from build123d import *

# Parameters (mm, degrees)
CROQUIS1_R                 = 7.5
SALIENTE_EXTRUIR1_DEPTH    = 10
C_PULA1_FACE_RADIUS        = 7.5
C_PULA1_HEIGHT             = 7.5
CORTAR_EXTRUIR1_DEPTH      = 10
CORTAR_EXTRUIR1_DEPTH_BACK = 19
CORTAR_EXTRUIR2_DEPTH      = 11
CORTAR_EXTRUIR2_DEPTH_BACK = 19
CROQUIS3_R                 = 1.25
REDONDEO1_R                = 0.5


with BuildPart() as part:
    # Croquis1 → Saliente-Extruir1 (new body)
    with BuildSketch(Plane.XY):
        Circle(CROQUIS1_R)
    extrude(amount=SALIENTE_EXTRUIR1_DEPTH)

    # Cúpula1: a dome of height H over a round flat face of radius A is a cap of a sphere of radius (A * A + H * H) / (2 * H)
    c_pula1_r = (C_PULA1_FACE_RADIUS * C_PULA1_FACE_RADIUS + C_PULA1_HEIGHT * C_PULA1_HEIGHT) / (2 * C_PULA1_HEIGHT)
    c_pula1_base = Plane((0, 0, 10), z_dir=(0, 0, 1))
    with Locations(c_pula1_base.offset(C_PULA1_HEIGHT - c_pula1_r)):
        c_pula1_ball = Sphere(c_pula1_r, mode=Mode.PRIVATE)
    add(split(c_pula1_ball, bisect_by=c_pula1_base, keep=Keep.TOP, mode=Mode.PRIVATE))

    # Croquis2 → Cortar-Extruir1 (cut, two sides: drawn at the far end of the back side and taken through both)
    with BuildSketch(Plane(origin=(0, 0, 0), x_dir=(1, 0, 0), z_dir=(0, 1, 0)).offset(-CORTAR_EXTRUIR1_DEPTH_BACK)):
        Polygon((-4, -10), (-4, -17.5), (4, -17.5), (4, -9.5), (4, -5), (-4, -5), align=None)
    extrude(amount=CORTAR_EXTRUIR1_DEPTH + CORTAR_EXTRUIR1_DEPTH_BACK, mode=Mode.SUBTRACT)

    # Croquis3 → Cortar-Extruir2 (cut, two sides: drawn at the far end of the back side and taken through both)
    with BuildSketch(Plane(origin=(0, 0, 0), x_dir=(0, 0, -1), z_dir=(1, 0, 0)).offset(-CORTAR_EXTRUIR2_DEPTH_BACK)):
        with Locations(Location((-10, 0, 0), (0, 0, 270))):
            Circle(CROQUIS3_R)
    extrude(amount=CORTAR_EXTRUIR2_DEPTH + CORTAR_EXTRUIR2_DEPTH_BACK, mode=Mode.SUBTRACT)

    # Redondeo1
    # the kernel refuses this fillet: 0.5 mm, written as the material it takes off along each edge
    with BuildSketch(Plane(origin=(0, 0, 5), x_dir=(-0.6663010614300323, 0.7456828384354923, 0), z_dir=(-0.7456828384354923, -0.6663010614300323, 0))) as redondeo1_piece_1_section:
        with BuildLine():
            CenterArc((7.5 - REDONDEO1_R, REDONDEO1_R), REDONDEO1_R, 270, 90)
            Line((7.5 - REDONDEO1_R, 0), (7.5, 0))
            Line((7.5, 0), (7.5, REDONDEO1_R))
        make_face()
    redondeo1_piece_1 = revolve(axis=Axis((0, 0, 5), (0, 0, -1)), revolution_arc=83.564433706, mode=Mode.PRIVATE)
    redondeo1_piece_1 = split(redondeo1_piece_1, bisect_by=Plane(origin=(4, 7.359307854, 4.859307854), z_dir=(-1, 0, 0)), keep=Keep.TOP, mode=Mode.PRIVATE)
    redondeo1_piece_1 = split(redondeo1_piece_1, bisect_by=Plane(origin=(-4, 7.359307854, 4.859307854), z_dir=(1, 0, 0)), keep=Keep.TOP, mode=Mode.PRIVATE)
    add(redondeo1_piece_1, mode=Mode.SUBTRACT)
    with BuildSketch(Plane(origin=(4, -6.34428877, 10), x_dir=(0.807803952835934, 0.5894512480117758, 0), z_dir=(0, 0, -1)), Plane(origin=(-4, 6.34428877, 10), x_dir=(-0.8078039528359331, -0.5894512480117771, 0), z_dir=(0, 0, -1))) as redondeo1_piece_2:
        with BuildLine():
            CenterArc((0.982970703, -0.498849769), REDONDEO1_R, 86.112875875, 130.005200885)
            Line((0.579068726, -0.793575393), (0, 0))
            ThreePointArc((0, 0), (0.508433122, 0.017253461), (1.016866244, 0))
        make_face()
    extrude(amount=5, mode=Mode.SUBTRACT)
    with BuildSketch(Plane(origin=(4, 6.34428877, 10), x_dir=(0.8078039528359339, -0.5894512480117758, 0), z_dir=(0, 0, -1)), Plane(origin=(-4, -6.34428877, 10), x_dir=(-0.8078039528359333, 0.5894512480117767, 0), z_dir=(0, 0, -1))) as redondeo1_piece_3:
        with BuildLine():
            CenterArc((0.982970703, 0.498849769), REDONDEO1_R, 143.88192324, 130.005200885)
            Line((0.579068726, 0.793575393), (0, 0))
            ThreePointArc((0, 0), (0.508433122, -0.017253461), (1.016866244, 0))
        make_face()
    extrude(amount=5, mode=Mode.SUBTRACT)
    with BuildSketch(Plane(origin=(-4, 0, 10), x_dir=(0, 1, 0), z_dir=(0, 0, -1))) as redondeo1_piece_4:
        with BuildLine():
            CenterArc((5.361902647, -0.5), REDONDEO1_R, 319.994799115, 130.005200885)
            ThreePointArc((5.744895694, -0.821428571), (6.058529646, -0.42088436), (6.34428877, 0))
            Line((6.34428877, 0), (5.361902647, 0))
        make_face()
    revolve(axis=Axis((-4, 0, 10), (1, 0, 0)), revolution_arc=180, mode=Mode.SUBTRACT)
    with BuildSketch(Plane(origin=(4, 0, 10), x_dir=(0, 1, 0), z_dir=(0, 0, -1))) as redondeo1_piece_5:
        with BuildLine():
            CenterArc((5.361902647, 0.5), REDONDEO1_R, 270, 130.005200885)
            Line((5.361902647, 0), (6.34428877, 0))
            ThreePointArc((6.34428877, 0), (6.058529646, 0.42088436), (5.744895694, 0.821428571))
        make_face()
    revolve(axis=Axis((4, 0, 10), (1, 0, 0)), revolution_arc=180, mode=Mode.SUBTRACT)
    with BuildSketch(Plane(origin=(0, 0, 5), x_dir=(0.6663010614300334, -0.7456828384354912, 0), z_dir=(0.7456828384354912, 0.6663010614300334, 0))) as redondeo1_piece_6_section:
        with BuildLine():
            CenterArc((7.5 - REDONDEO1_R, REDONDEO1_R), REDONDEO1_R, 270, 90)
            Line((7.5 - REDONDEO1_R, 0), (7.5, 0))
            Line((7.5, 0), (7.5, REDONDEO1_R))
        make_face()
    redondeo1_piece_6 = revolve(axis=Axis((0, 0, 5), (0, 0, -1)), revolution_arc=83.564433706, mode=Mode.PRIVATE)
    redondeo1_piece_6 = split(redondeo1_piece_6, bisect_by=Plane(origin=(4, -7.359307854, 4.859307854), z_dir=(-1, 0, 0)), keep=Keep.TOP, mode=Mode.PRIVATE)
    redondeo1_piece_6 = split(redondeo1_piece_6, bisect_by=Plane(origin=(-4, -7.359307854, 4.859307854), z_dir=(1, 0, 0)), keep=Keep.TOP, mode=Mode.PRIVATE)
    add(redondeo1_piece_6, mode=Mode.SUBTRACT)
    with BuildSketch(Plane(origin=(-4, 6.34428877, 10), x_dir=(-0.8078039528359331, -0.5894512480117771, 0), z_dir=(0, 0, -1))) as redondeo1_piece_7a_section:
        with BuildLine():
            CenterArc((0.982970703, -0.498849769), REDONDEO1_R, 86.112875875, 130.005200885)
            Line((0.579068726, -0.793575393), (0, 0))
            ThreePointArc((0, 0), (0.508433122, 0.017253461), (1.016866244, 0))
        make_face()
    redondeo1_piece_7a = extrude(amount=7.54216561, mode=Mode.PRIVATE)
    redondeo1_piece_7a = split(redondeo1_piece_7a, bisect_by=Plane(origin=(-4.209576919, 5.957871406, 5), z_dir=(0, 0, -1)), keep=Keep.TOP, mode=Mode.PRIVATE)
    with BuildSketch(Plane(origin=(0, 0, 5), x_dir=(-0.6663010614300323, 0.7456828384354923, 0), z_dir=(-0.7456828384354923, -0.6663010614300323, 0))) as redondeo1_piece_7b_section:
        with BuildLine():
            CenterArc((7.5 - REDONDEO1_R, REDONDEO1_R), REDONDEO1_R, 270, 90)
            Line((7.5 - REDONDEO1_R, 0), (7.5, 0))
            Line((7.5, 0), (7.5, REDONDEO1_R))
        make_face()
    redondeo1_piece_7b = revolve(axis=Axis((0, 0, 5), (0, 0, -1)), revolution_arc=83.564433706, mode=Mode.PRIVATE)
    redondeo1_piece_7b = split(redondeo1_piece_7b, bisect_by=Plane(origin=(-4, 5.878976183, 4.882052038), z_dir=(-1, 0, 0)), keep=Keep.TOP, mode=Mode.PRIVATE)
    redondeo1_piece_7 = redondeo1_piece_7a & redondeo1_piece_7b
    add(redondeo1_piece_7, mode=Mode.SUBTRACT)
    with BuildSketch(Plane(origin=(0, 0, 5), x_dir=(-0.6663010614300323, 0.7456828384354923, 0), z_dir=(-0.7456828384354923, -0.6663010614300323, 0))) as redondeo1_piece_8a_section:
        with BuildLine():
            CenterArc((7.5 - REDONDEO1_R, REDONDEO1_R), REDONDEO1_R, 270, 90)
            Line((7.5 - REDONDEO1_R, 0), (7.5, 0))
            Line((7.5, 0), (7.5, REDONDEO1_R))
        make_face()
    redondeo1_piece_8a = revolve(axis=Axis((0, 0, 5), (0, 0, -1)), revolution_arc=83.564433706, mode=Mode.PRIVATE)
    redondeo1_piece_8a = split(redondeo1_piece_8a, bisect_by=Plane(origin=(4, 5.878976375, 4.882052003), z_dir=(1, 0, 0)), keep=Keep.TOP, mode=Mode.PRIVATE)
    with BuildSketch(Plane(origin=(4, 6.34428877, 10), x_dir=(0.8078039528359339, -0.5894512480117758, 0), z_dir=(0, 0, -1))) as redondeo1_piece_8b_section:
        with BuildLine():
            CenterArc((0.982970703, 0.498849769), REDONDEO1_R, 143.88192324, 130.005200885)
            Line((0.579068726, 0.793575393), (0, 0))
            ThreePointArc((0, 0), (0.508433122, -0.017253461), (1.016866244, 0))
        make_face()
    redondeo1_piece_8b = extrude(amount=7.54216561, mode=Mode.PRIVATE)
    redondeo1_piece_8b = split(redondeo1_piece_8b, bisect_by=Plane(origin=(4.209576919, 5.957871406, 5), z_dir=(0, 0, -1)), keep=Keep.TOP, mode=Mode.PRIVATE)
    redondeo1_piece_8 = redondeo1_piece_8a & redondeo1_piece_8b
    add(redondeo1_piece_8, mode=Mode.SUBTRACT)
    with BuildSketch(Plane(origin=(4, -6.34428877, 10), x_dir=(0.807803952835934, 0.5894512480117758, 0), z_dir=(0, 0, -1))) as redondeo1_piece_9a_section:
        with BuildLine():
            CenterArc((0.982970703, -0.498849769), REDONDEO1_R, 86.112875875, 130.005200885)
            Line((0.579068726, -0.793575393), (0, 0))
            ThreePointArc((0, 0), (0.508433122, 0.017253461), (1.016866244, 0))
        make_face()
    redondeo1_piece_9a = extrude(amount=7.54216561, mode=Mode.PRIVATE)
    redondeo1_piece_9a = split(redondeo1_piece_9a, bisect_by=Plane(origin=(4.209576919, -5.957871406, 5), z_dir=(0, 0, -1)), keep=Keep.TOP, mode=Mode.PRIVATE)
    with BuildSketch(Plane(origin=(0, 0, 5), x_dir=(0.6663010614300334, -0.7456828384354912, 0), z_dir=(0.7456828384354912, 0.6663010614300334, 0))) as redondeo1_piece_9b_section:
        with BuildLine():
            CenterArc((7.5 - REDONDEO1_R, REDONDEO1_R), REDONDEO1_R, 270, 90)
            Line((7.5 - REDONDEO1_R, 0), (7.5, 0))
            Line((7.5, 0), (7.5, REDONDEO1_R))
        make_face()
    redondeo1_piece_9b = revolve(axis=Axis((0, 0, 5), (0, 0, -1)), revolution_arc=83.564433706, mode=Mode.PRIVATE)
    redondeo1_piece_9b = split(redondeo1_piece_9b, bisect_by=Plane(origin=(4, -5.878976176, 4.88205204), z_dir=(1, 0, 0)), keep=Keep.TOP, mode=Mode.PRIVATE)
    redondeo1_piece_9 = redondeo1_piece_9a & redondeo1_piece_9b
    add(redondeo1_piece_9, mode=Mode.SUBTRACT)
    with BuildSketch(Plane(origin=(0, 0, 5), x_dir=(0.6663010614300334, -0.7456828384354912, 0), z_dir=(0.7456828384354912, 0.6663010614300334, 0))) as redondeo1_piece_10a_section:
        with BuildLine():
            CenterArc((7.5 - REDONDEO1_R, REDONDEO1_R), REDONDEO1_R, 270, 90)
            Line((7.5 - REDONDEO1_R, 0), (7.5, 0))
            Line((7.5, 0), (7.5, REDONDEO1_R))
        make_face()
    redondeo1_piece_10a = revolve(axis=Axis((0, 0, 5), (0, 0, -1)), revolution_arc=83.564433706, mode=Mode.PRIVATE)
    redondeo1_piece_10a = split(redondeo1_piece_10a, bisect_by=Plane(origin=(-4, -5.878976383, 4.882052), z_dir=(-1, 0, 0)), keep=Keep.TOP, mode=Mode.PRIVATE)
    with BuildSketch(Plane(origin=(-4, -6.34428877, 10), x_dir=(-0.8078039528359333, 0.5894512480117767, 0), z_dir=(0, 0, -1))) as redondeo1_piece_10b_section:
        with BuildLine():
            CenterArc((0.982970703, 0.498849769), REDONDEO1_R, 143.88192324, 130.005200885)
            Line((0.579068726, 0.793575393), (0, 0))
            ThreePointArc((0, 0), (0.508433122, -0.017253461), (1.016866244, 0))
        make_face()
    redondeo1_piece_10b = extrude(amount=7.54216561, mode=Mode.PRIVATE)
    redondeo1_piece_10b = split(redondeo1_piece_10b, bisect_by=Plane(origin=(-4.209576919, -5.957871406, 5), z_dir=(0, 0, -1)), keep=Keep.TOP, mode=Mode.PRIVATE)
    redondeo1_piece_10 = redondeo1_piece_10a & redondeo1_piece_10b
    add(redondeo1_piece_10, mode=Mode.SUBTRACT)


solid = part.part
The listing builds one solid part. Answer for the finished solid, in the listing's coordinates (mm). A direction names the side the tool comes from. Round coordinates to 2 decimals unless told otherwise and drop trailing zeros. Order: outer loops, then holes, each group sorted by start corner. A loop starts at its lowest first (then second) coordinate and runs counter-clockwise, first axis right, second up. Notation, with made-up numbers: (13.25, 36) -> (72.25, 36) arc R13 ccw to (72.25, 52) -> close; hole circle Ø5 at (86, 73.25). An arc over 180 degrees is marked (long way). One line per item, written item: value.
Item 1: Given P1, Ø1.5, axis at x = 6, z = 14, coming from the -Y side; P2, Ø5, axis at x = 3, z = 12, coming from the -Y side; P3, Ø2.5, axis at x = -1, y = 0.5, coming from the +Z side, each flat-ended and moving along its own axis, determine where each tip first touches the part or whether it passes through.
Taken from the geometry:
P1: stops at y = -3.81
P2: stops at y = -5.86
P3: stops at z = 5
Item 2: Find section D-D, the plane x = 0. Give the vertices of the cut face in (y, z), then the cut area to 3 significant figures.
Taken from the geometry:
outline: (-7.5, 0) -> (7.5, 0) -> (7.5, 4.5) arc R0.5 ccw to (7, 5) -> (-7, 5) arc R0.5 ccw to (-7.5, 4.5) -> close
area: 74.9 mm2
Item 3: Find section B-B, the plane y = 0. Give the vertices of the cut face in (x, z).
Taken from the geometry:
outline: (-7.5, 0) -> (7.5, 0) -> (7.5, 8.75) -> (4, 8.75) -> (4, 5) -> (-4, 5) -> (-4, 8.75) -> (-7.5, 8.75) -> close; (-7.4, 11.25) -> (-4, 11.25) -> (-4, 15.36) arc R0.5 ccw to (-4.82, 15.74) arc R7.5 ccw to start; (4, 11.25) -> (7.4, 11.25) arc R7.5 ccw to (4.82, 15.74) arc R0.5 ccw to (4, 15.36) -> close
Item 4: For a pull along X with two mould halves and no side action, classify faces 1 (the cylindrical face through (-5.776, -0.672, 8.946)), 2 (the cylindrical face through (4.3, -5.82, 7.29)), 3 (the cylindrical face through (-7.493, 0.33, 3.819)) as released by +X, released by -X, zero draft, split by the parting line, or undercut.
Taken from the geometry:
face 1: zero draft
face 2: undercut
face 3: split by the parting line
Item 5: Straight lines are drawn through the part: L1, parallel to X at y = -1.25, z = 7; L2, parallel to Y at x = -5.65, z = 10; L3, parallel to Z at x = 0.75, y = -2.5. For each, find the intervals that lie inside material, in ascending order.
Taken from the geometry:
L1: x = -7.4 to -4, 4 to 7.4
L2: y = -4.93 to -1.25, 1.25 to 4.93
L3: z = 0 to 5
Item 6: Find section A-A, the plane z = 7.75. Give the vertices of the cut face in (x, y).
Taken from the geometry:
outline: (-4.82, -5.74) arc R0.5 ccw to (-4, -5.36) -> (-4, 5.36) arc R0.5 ccw to (-4.82, 5.74) arc R7.5 ccw to start; (4, -5.36) arc R0.5 ccw to (4.82, -5.74) arc R7.5 ccw to (4.82, 5.74) arc R0.5 ccw to (4, 5.36) -> close
Item 7: For faces 4 (the cylindrical face through (5.73, 0.16, 8.76)), 5 (the cylindrical face through (-4.28, -5.81, 7.29)), 6 (the flat face through (4, 1, 9)), 7 (the cylindrical face through (-4.3, 5.82, 7.29)), determine the directions among +Z, -Z, +X, -X, +Y, -Y from which every point of the face is accessible in a straight line to the end or side of a thin tool.
Taken from the geometry:
face 4: +X, -X
face 5: +Z, -Y
face 6: +Z, +Y, -Y
face 7: +Z, +Y
Item 8: Find section C-C, the plane x = 6. Give the vertices of the cut face in (y, z), then the cut area to 3 significant figures.
Taken from the geometry:
outline: (-4.5, 0) -> (4.5, 0) -> (4.5, 10) arc R4.5 ccw to (-4.5, 10) -> close; hole circle Ø2.5 at (0, 10)
area: 117 mm2
